Geometry check sheet. Reference: the model listing, model coordinates, mm. A direction names the side the tool comes from. Round coordinates to 2 decimals unless told otherwise and drop trailing zeros. Write each loop counter-clockwise with the first axis right and the second up, starting at its lowest first coordinate (ties: lowest second). Pieces come first, ordered by that corner, then holes. Notation, with made-up numbers: M -25,88.25 L 12,88.25 A18 ccw 12,115.25 Z; hole C 49.25,50 d3. An arc over 180 degrees is marked long. Answer in a Markdown table with one row per item. Add a question column.
from build123d import *

# Parameters (mm, degrees)
BOSS_EXTRUDE1_DEPTH = 25
CHAMFER1_SIZE       = 8
CHAMFER2_SIZE       = 3
CHAMFER3_SIZE       = 4
CHAMFER4_SIZE       = 2


with BuildPart() as part:
    # Sketch1 → Boss-Extrude1 (new body)
    with BuildSketch(Plane(origin=(0, 0, 0), x_dir=(0, 0, -1), z_dir=(1, 0, 0))):
        Polygon((-10.227272727, 11.022727273), (-7.227272727, 11.022727273), (-7.227272727, -43.977272727), (24.772727273, -43.977272727), (24.772727273, -33.977272727), (27.772727273, -33.977272727), (27.772727273, -43.977272727), (27.772727273, -48.977272727), (-7.227272727, -48.977272727), (-10.227272727, -48.977272727), align=None)
    extrude(amount=BOSS_EXTRUDE1_DEPTH)

    # Chamfer1
    chamfer1_edges = [part.edges().sort_by_distance(p)[0] for p in [
        (12.5, -43.977272727, 7.227272727),
    ]]
    chamfer(chamfer1_edges, length=CHAMFER1_SIZE)

    # Chamfer2
    chamfer2_edges = [part.edges().sort_by_distance(p)[0] for p in [
        (12.5, -43.977272727, -24.772727273),
        (12.5, -48.977272727, 10.227272727),
    ]]
    chamfer(chamfer2_edges, length=CHAMFER2_SIZE)

    # Chamfer3
    chamfer3_edges = [part.edges().sort_by_distance(p)[0] for p in [
        (12.5, -48.977272727, -27.772727273),
    ]]
    chamfer(chamfer3_edges, length=CHAMFER3_SIZE)

    # Chamfer4
    chamfer4_edges = [part.edges().sort_by_distance(p)[0] for p in [
        (12.5, -33.977272727, -27.772727273),
    ]]
    chamfer(chamfer4_edges, length=CHAMFER4_SIZE)


solid = part.part
Item 1: Gauge pin test, flat ends, axial feed: pin 1 Ø10 at (x, y) = (14, -13) entering from -Z; pin 2 Ø0.8 at (x, z) = (17.5, -25.5) entering from +Y; pin 3 Ø8 at (x, z) = (3, -18) entering from +Y. Record the tip position at first contact, or that the pin passes through.
Item 2: Scan lines: probe 1 along Y at (x, z) = (15, -1.5); probe 2 along Z at (x, y) = (20, -42); probe 3 along Z at (x, y) = (17.75, -30). Record each from-to range of solid material in increasing order. Write a range as from..to.
Item 3: Access from +Z, -Z, +X, -X, +Y, -Y to the whole of each face (thin tool, end or side, straight path). Record for faces 1 (the flat face through (12, -38, -24.773)), 2 (the flat face through (12, -18, 10.227)).
Item 4: Mould release check, pull along Z, two halves, no side actions. Record for faces 3 (the flat face through (12.32, -42.46, -23.29)), 4 (the flat face through (12, -48.977, -8)), 5 (the flat face through (12.33, -47.01, -25.74)): +Z half, -Z half, draft (parallel to the pull), parting line (faces both ways), or undercut.
Item 5: Section check A-A, the plane x = 13.25. Record the boundary of the cut face in (y, z).
Item 6: Section check C-C, the plane z = -3. Record the boundary of the cut face in (x, y), and give its area (3 significant figures).
Item 7: Section check B-B, the plane y = 0. Record the boundary of the cut face in (x, z), and give its area (3 significant figures).
Result sheet:
| question | item | result |
|---|---|---|
| 1 | pin 1 | stops at z = 7.23 |
| 1 | pin 2 | stops at y = -33.98 |
| 1 | pin 3 | stops at y = -43.75 |
| 2 | probe 1 | y = -48.98..-43.98 |
| 2 | probe 2 | z = -27.77..-23.75, 1.2..10.23 |
| 2 | probe 3 | z = 7.23..10.23 |
| 3 | face 1 | +X, -X, +Y |
| 3 | face 2 | +Z, +X, -X, +Y, -Y |
| 4 | face 3 | undercut |
| 4 | face 4 | draft |
| 4 | face 5 | -Z half |
| 5 | outline | M -48.98,-23.77 L -44.98,-27.77 L -35.98,-27.77 L -33.98,-25.77 L -33.98,-24.77 L -40.98,-24.77 L -43.98,-21.77 L -43.98,-0.77 L -35.98,7.23 L 11.02,7.23 L 11.02,10.23 L -45.98,10.23 L -48.98,7.23 Z |
| 6 | outline | M 0,-48.98 L 25,-48.98 L 25,-43.98 L 0,-43.98 Z |
| 6 | area | 125 mm^2 |
| 7 | outline | M 0,7.23 L 25,7.23 L 25,10.23 L 0,10.23 Z |
| 7 | area | 75.0 mm^2 |
